```python
from build123d import *

# Parameters (mm, degrees)
BOSS_EXTRUDE1_DEPTH = 30


with BuildPart() as part:
    # Sketch1 → Boss-Extrude1 (new body)
    with BuildSketch(Plane(origin=(0, 7.5, 0), x_dir=(1, 0, 0), z_dir=(0, 1, 0))):
        with BuildLine():
            Line((248.792121733, 471.76093065), (217.679423361, 502.873629023))
            Line((217.679423361, 502.873629023), (214.850996236, 500.045201898))
            Line((214.850996236, 500.045201898), (243.135267484, 471.76093065))
            ThreePointArc((243.135267484, 471.76093065), (244.599733578, 468.225396744), (243.135267484, 464.689862838))
            Line((243.135267484, 464.689862838), (191.566724989, 413.121320344))
            ThreePointArc((191.566724989, 413.121320344), (190.482861232, 411.499203599), (190.102258895, 409.585786438))
            Line((190.102258895, 409.585786438), (190.102258895, 376.656854249))
            Line((190.102258895, 376.656854249), (194.102258895, 376.656854249))
            Line((194.102258895, 376.656854249), (194.102258895, 407.928932188))
            ThreePointArc((194.102258895, 407.928932188), (194.482861232, 409.84234935), (195.566724989, 411.464466094))
            Line((195.566724989, 411.464466094), (248.792121733, 464.689862838))
            ThreePointArc((248.792121733, 464.689862838), (250.256587827, 468.225396744), (248.792121733, 471.76093065))
        make_face()
    extrude(amount=-BOSS_EXTRUDE1_DEPTH)


solid = part.part
```
Geometry: final body of the model. Coordinates: model frame, mm. A direction names the side the tool comes from. Round coordinates to 2 decimals unless told otherwise and drop trailing zeros. Order: outer loops, then holes, each group sorted by start corner. A loop starts at its lowest first (then second) coordinate and runs counter-clockwise, first axis right, second up. Notation, with made-up numbers: (5.25, 21.25) - (36.25, 21.25) arc R7 ccw to (36.25, 30.25) - close; hole circle Ø4 at (-20, 84). An arc over 180 degrees is marked (long way). Use CSV: the item, a comma, the result in double quotes. Start each with the question number.
Q1. Section query D-D (x = 216). Return loops of the section in (y, z), and give its area (3 significant figures).
Q2. Access query for faces 4 (the face through (194.102, -7, -392)), 5 (the face through (220, 7.5, -440)), 6 (the face through (228.795, -7.29, -486.101)). Directions: +Z, -Z, +X, -X, +Y, -Y. A direction counts if a zero-diameter tool reaches every point of the face in a straight line with its end or side. Return the directions, or none.
Q3. First-contact query: pin 1 (8 mm diameter, centred on x = 228.5, y = -2.5, fed in from +Z); pin 2 (8 mm diameter, centred on x = 203.5, z = -429, fed in from +Y); pin 3 (12 mm diameter, centred on y = -19.5, z = -480.5, fed in from +X); pin 4 (12 mm diameter, centred on x = 219.5, y = 2, fed in from +Z). Flat tips, straight axial feed; report the tip coordinate or a pass-through.
Q4. Material intervals for line 1 along X through (y, z) = (-20.25, -406.5); line 2 along Z through (x, y) = (215.5, -18.75); line 3 along Z through (x, y) = (217.5, -6.5), sorted ascending. Write a range as from..to.
Q5. Section query A-A (x = 225). Return loops of the section in (y, z), and give its area (3 significant figures).
Q6. Mould query, pull axis Z, two halves, no side actions, for faces 1 (the face through (250.256, -7.29, -468.17)), 2 (the face through (244.6, -7.3, -468.3)), 3 (the face through (194.472, -7.29, -409.817)). Classes: +Z half, -Z half, draft (parallel to the pull), parting line (faces both ways), or undercut.
Q7. Section query B-B (y = -2.25). Return loops of the section in (x, z), and give its area (3 significant figures).
Q8. Section query C-C (z = -389). Return loops of the section in (x, y), and give its area (3 significant figures).
Result set:
1,outline,"(-22.5, -501.19) - (7.5, -501.19) - (7.5, -498.9) - (-22.5, -498.9) - close; (-22.5, -437.55) - (7.5, -437.55) - (7.5, -431.9) - (-22.5, -431.9) - close"
1,area,"239 mm2"
2,face 4,"+Z, +X, +Y, -Y"
2,face 5,"+Z, -Z, +X, -X, +Y"
2,face 6,"-X, +Y, -Y"
3,pin 1,"stops at z = -440.4"
3,pin 2,"stops at y = 7.5"
3,pin 3,"stops at x = 246.05"
3,pin 4,"stops at z = -429.4"
4,line 1,"x = 190.1..194.1"
4,line 2,"z = -500.69..-499.4, -437.05..-431.4"
4,line 3,"z = -502.69..-497.4, -439.05..-433.4"
5,outline,"(-22.5, -495.55) - (7.5, -495.55) - (7.5, -489.9) - (-22.5, -489.9) - close; (-22.5, -446.55) - (7.5, -446.55) - (7.5, -440.9) - (-22.5, -440.9) - close"
5,area,"339 mm2"
6,face 1,"parting line"
6,face 2,"undercut"
6,face 3,"+Z half"
7,outline,"(190.1, -409.59) arc R5 ccw to (191.57, -413.12) - (243.14, -464.69) arc R5 cw to (243.14, -471.76) - (214.85, -500.05) - (217.68, -502.87) - (248.79, -471.76) arc R5 ccw to (248.79, -464.69) - (195.57, -411.46) arc R5 cw to (194.1, -407.93) - (194.1, -376.66) - (190.1, -376.66) - close"
7,area,"649 mm2"
8,outline,"(190.1, -22.5) - (194.1, -22.5) - (194.1, 7.5) - (190.1, 7.5) - close"
8,area,"120 mm2"
